from build123d import *

# Parameters (mm, degrees)
SKETCH1_R           = 3
BOSS_EXTRUDE1_DEPTH = 2
SKETCH2_W           = 2
SKETCH2_H           = 9
BOSS_EXTRUDE2_DEPTH = 75
FILLET1_R           = 2


with BuildPart() as part:
    # Sketch1 → Boss-Extrude1 (new body)
    with BuildSketch(Plane.XY):
        with BuildLine():
            Line((-7.5, 4.5), (2, 4.5))
            ThreePointArc((2, 4.5), (3.414213562, 3.914213562), (4, 2.5))
            Line((4, 2.5), (4, -2.5))
            ThreePointArc((4, -2.5), (3.414213562, -3.914213562), (2, -4.5))
            Line((2, -4.5), (-7.5, -4.5))
            Line((-7.5, -4.5), (-7.5, 4.5))
        make_face()
        Circle(SKETCH1_R, mode=Mode.SUBTRACT)
    extrude(amount=BOSS_EXTRUDE1_DEPTH)

    # Sketch2 → Boss-Extrude2 (add)
    with BuildSketch(Plane(origin=(0, 0, 0), x_dir=(-1, 0, 0), z_dir=(0, 0, -1))):
        with Locations((6.5, 0)):
            Rectangle(SKETCH2_W, SKETCH2_H)
    extrude(amount=BOSS_EXTRUDE2_DEPTH)

    # Fillet1
    fillet1_edges = [part.edges().sort_by_distance(p)[0] for p in [
        (-5.5, 0, 0),
        (-7.5, 0, 2),
    ]]
    fillet(fillet1_edges, radius=FILLET1_R)


solid = part.part
Verification items for the finished model (mm, model axes). A direction names the side the tool comes from. Give positions to 0.01 mm unless a question says otherwise; leave off trailing zeros. Write each loop counter-clockwise with the first axis right and the second up, starting at its lowest first coordinate (ties: lowest second). Pieces come first, ordered by that corner, then holes. Notation, with made-up numbers: M 0,55.5 L 57,55.5 A21 cw 57,59.5 Z; hole C 86,34 d7. An arc over 180 degrees is marked long. Put each result on its own line as item: value. Start each with the question number.
1. Section check A-A (x = 0). Record the cut outline in (y, z), and give its area (3 significant figures).
2. Scan lines: line 1 along Y through (x, z) = (0, 1.4); line 2 along X through (y, z) = (1.25, -41); line 3 along Z through (x, y) = (3.75, -0.5). Record each from-to range of solid material in increasing order. Write a range as [from, to].
3. Section check B-B (y = 0). Record the cut outline in (x, z), and give its area (3 significant figures).
4. Draft check along Y on faces 1 (the face through (-6.93, 0.06, 1.4)), 2 (the face through (3.43, -3.9, 0.99)), 3 (the face through (-3, 0, 1)). Enter one of: +Y half, -Y half, draft (parallel to the pull), parting line (faces both ways), or undercut.
5. Go/stop test with flat-tipped pins: pin 1 Ø6 at (x, z) = (-4, -16) entering from +Y; pin 2 Ø1.5 at (x, y) = (0, -1.5) entering from -Z. Record where each tip stops, or that it passes through.
6. Section check C-C (z = -38). Record the cut outline in (x, y).
7. Set-up check for faces 4 (the face through (-3, 2, 2)), 5 (the face through (-5.5, 0, -38)): record each of +Z, -Z, +X, -X, +Y, -Y from which the full face is reachable in a straight line by a thin tool's end or side.
Answer list:
1. outline: M -4.5,0 L -3,0 L -3,2 L -4.5,2 Z; M 3,0 L 4.5,0 L 4.5,2 L 3,2 Z
1. area: 6.00 mm2
2. line 1: [-4.5, -3], [3, 4.5]
2. line 2: [-7.5, -5.5]
2. line 3: [0, 2]
3. outline: M -7.5,-75 L -5.5,-75 L -5.5,-2 A2 cw -3.5,0 L -3,0 L -3,2 L -5.5,2 A2 ccw -7.5,0 Z; M 3,0 L 4,0 L 4,2 L 3,2 Z
3. area: 161 mm2
4. face 1: draft
4. face 2: -Y half
4. face 3: undercut
5. pin 1: y = 4.5
5. pin 2: through
6. outline: M -7.5,-4.5 L -5.5,-4.5 L -5.5,4.5 L -7.5,4.5 Z
7. face 4: +Z, +X, -X, +Y, -Y
7. face 5: -Z, +X, +Y, -Y
